Part model, mm, in its own coordinate system. A direction names the side the tool comes from. Coordinates: 2 decimals unless noted, no trailing zeros. Write each loop counter-clockwise with the first axis right and the second up, starting at its lowest first coordinate (ties: lowest second). Pieces come first, ordered by that corner, then holes. Notation, with made-up numbers: (-33, 12) - (-25, 12) arc R9 ccw to (-25, 16) - close; hole circle Ø6 at (-20, -8). An arc over 180 degrees is marked (long way). Use a Markdown table: item, result.
```python
from build123d import *

# Parameters (mm, degrees)
SKETCH1_W           = 1
SKETCH1_H           = 1
BOSS_EXTRUDE1_DEPTH = 14
FILLET1_R           = 0.5


with BuildPart() as part:
    # Sketch1 → Boss-Extrude1 (new body)
    with BuildSketch(Plane.XY):
        Polygon((0, 4.925), (-3.7, 4.925), (-3.7, 3.925), (-1.2, 3.925), (-1.2, 0), (0, 0), align=None)
        Polygon((0, -4.925), (0, 0), (-1.2, 0), (-1.2, -3.925), (-3.5, -3.925), (-4.5, -3.925), (-4.5, -4.925), align=None)
        with Locations((-4, -3.425)):
            Rectangle(SKETCH1_W, SKETCH1_H)
    extrude(amount=BOSS_EXTRUDE1_DEPTH)

    # Fillet1
    fillet1_edges = [part.edges().sort_by_distance(p)[0] for p in [
        (0, -4.925, 7),
        (-4.5, -4.925, 7),
        (-4.5, -2.925, 7),
        (-3.5, -2.925, 7),
        (-3.7, 3.925, 7),
        (-3.7, 4.925, 7),
        (0, 4.925, 7),
    ]]
    fillet(fillet1_edges, radius=FILLET1_R - 0.0001)  # a hair under: the kernel refuses the full size


solid = part.part
```
Item 1: Drop a flat-ended pin along its axis: P1, Ø2, axis at x = -3.5, y = 1, coming from the -Z side. Give the stop position or say it passes through.
From the geometry:
| item | result |
|---|---|
| P1 | through |
Item 2: Band-saw the part on D-D, the plane x = -3.85. Give the cut face in (y, z) (3 decimals).
From the geometry:
| item | result |
|---|---|
| outline | (-4.925, 0) - (-2.948, 0) - (-2.948, 14) - (-4.925, 14) - close |
Item 3: Drill centre lines: probe 1 along Y at (x, z) = (-1.25, 6.5) (3 decimals); probe 2 along X at (y, z) = (-3.5, 3.5); probe 3 along X at (y, z) = (-1.5, 4.75). Where is each one in solid material? Low to high.
From the geometry:
| item | result |
|---|---|
| probe 1 | -4.925 to -3.925, 3.925 to 4.925 |
| probe 2 | -4.5 to -3.5, -1.2 to 0 |
| probe 3 | -1.2 to 0 |
Item 4: Two-plate mould, pull along Y, no slides. Class faces 1 (the face through (-1, 0, 14)), 2 (the face through (-2, 3.925, 7)), 3 (the face through (-2, 4.925, 7)): pulls with the +Y half, pulls with the -Y half, needs draft (parallel to the pull), parting line crosses it, or undercut.
From the geometry:
| item | result |
|---|---|
| face 1 | needs draft |
| face 2 | undercut |
| face 3 | pulls with the +Y half |
Item 5: Which spindle directions (+Z, -Z, +X, -X, +Y, -Y) get a long thin tool onto all of the face, cutting with end or side? Do faces 4 (the face through (-4.5, -4, 7)), 5 (the face through (-2, -3.925, 7)). Say none if no direction does.
From the geometry:
| item | result |
|---|---|
| face 4 | +Z, -Z, -X, +Y, -Y |
| face 5 | +Z, -Z |
Item 6: Band-saw the part on C-C, the plane y = 1.5. Give the cut face in (x, z).
From the geometry:
| item | result |
|---|---|
| outline | (-1.2, 0) - (0, 0) - (0, 14) - (-1.2, 14) - close |
Item 7: Band-saw the part on A-A, the plane x = -1.35. Give the cut face in (y, z) (3 decimals).
From the geometry:
| item | result |
|---|---|
| outline | (-4.925, 0) - (-3.925, 0) - (-3.925, 14) - (-4.925, 14) - close; (3.925, 0) - (4.925, 0) - (4.925, 14) - (3.925, 14) - close |
